from build123d import *

# Parameters (mm, degrees)
ESBO_O1_W                = 103
ESBO_O1_H                = 34
RESSALTO_EXTRUS_O1_DEPTH = 24
CORTE_EXTRUS_O1_DEPTH    = 0.5
FILETE1_R                = 2
SKETCH1_R                = 2.5
BOSS_EXTRUDE1_DEPTH      = 2


with BuildPart() as part:
    # Esboço1 → Ressalto-extrusão1 (new body)
    with BuildSketch(Plane.XY):
        Rectangle(ESBO_O1_W, ESBO_O1_H)
    extrude(amount=RESSALTO_EXTRUS_O1_DEPTH)

    # Esboço2 → Corte-extrusão1 (cut)
    with BuildSketch(Plane(origin=(51.5, 0, 0), x_dir=(0, 0, -1), z_dir=(1, 0, 0))):
        with BuildLine():
            Line((-4.5, 6), (-4.5, -6))
            ThreePointArc((-4.5, -6), (-12, -13.5), (-19.5, -6))
            Line((-19.5, -6), (-19.5, 6))
            ThreePointArc((-19.5, 6), (-12, 13.5), (-4.5, 6))
        make_face()
    corte_extrus_o1 = extrude(amount=-CORTE_EXTRUS_O1_DEPTH, mode=Mode.SUBTRACT)

    # Espelhar1: Corte-extrusão1 across plane
    add(corte_extrus_o1.mirror(Plane(origin=(0, 0, 0), x_dir=(0, 0, 1), z_dir=(1, 0, 0))), mode=Mode.SUBTRACT)

    # Filete1
    filete1_edges = [part.edges().sort_by_distance(p)[0] for p in [
        (-51.5, 0, 24),
        (0, -17, 24),
        (51.5, 0, 24),
        (0, -17, 0),
        (-51.5, 0, 0),
        (0, 17, 0),
        (51.5, 0, 0),
        (0, 17, 24),
        (51.5, -17, 12),
        (-51.5, -17, 12),
        (-51.5, 17, 12),
        (51.5, 17, 12),
    ]]
    fillet(filete1_edges, radius=FILETE1_R)

    # Sketch1 → Boss-Extrude1 (add)
    with BuildSketch(Plane.XY.offset(24)):
        Circle(SKETCH1_R)
    extrude(amount=BOSS_EXTRUDE1_DEPTH)


solid = part.part
Check sheet for the modelled part. Datum: model origin and axes. Units: mm. A direction names the side the tool comes from. Give positions to 0.01 mm unless a question says otherwise; leave off trailing zeros. Order: outer loops, then holes, each group sorted by start corner. A loop starts at its lowest first (then second) coordinate and runs counter-clockwise, first axis right, second up. Notation, with made-up numbers: M 0.25,19 L 46.25,19 A16 ccw 46.25,43 Z; hole C -34,-14.75 d6. An arc over 180 degrees is marked long. Answer as CSV lines item,"result". Start each with the question number.
Item 1: Gauge pin test, flat ends, axial feed: P1, Ø8, axis at x = -4.5, y = -6.5, coming from the +Z side; P2, Ø0.6, axis at x = -51.5, y = -1.5, coming from the +Z side; P3, Ø1, axis at x = 4, z = 23, coming from the -Y side. Record the tip position at first contact, or that the pin passes through.
Item 2: Cross-section at B-B on y = 0. Enter the section's corners in (x, z), plus the area to 3 significant figures.
Item 3: Cross-section at C-C on y = 11. Enter the section's corners in (x, z).
Item 4: Thickness scan on line 1 (X direction, y = 0, z = 15.5); line 2 (Z direction, x = 45, y = -8); line 3 (X direction, y = -7, z = 1.75). Record the ranges inside material, lowest first. Write a range as [from, to].
Item 5: Cross-section at A-A on x = -24. Enter the section's corners in (y, z), plus the area to 3 significant figures.
Item 6: Tool access check on faces 1 (the face through (-51.25, -13.5, 11.84)), 2 (the face through (51, 0, 12)), 3 (the face through (-50.93, -16.4, 12.14)). Record the directions out of +Z, -Z, +X, -X, +Y, -Y that give a thin tool (end or side, any length) a straight path to the whole face; none if there is none.
Item 7: Mould release check, pull along Z, two halves, no side actions. Record for faces 4 (the face through (51.5, 0, 3)), 5 (the face through (51.25, 13.5, 12.16)), 6 (the face through (-50.93, 0.21, 0.6)): +Z half, -Z half, draft (parallel to the pull), parting line (faces both ways), or undercut.
Established:
1,P1,"stops at z = 24"
1,P2,"stops at z = 23.05"
1,P3,"stops at y = -16.94"
2,outline,"M -51.5,2 A2 ccw -49.5,0 L 49.5,0 A2 ccw 51.5,2 L 51.5,4.5 L 51,4.5 L 51,19.5 L 51.5,19.5 L 51.5,22 A2 ccw 49.5,24 L 2.5,24 L 2.5,26 L -2.5,26 L -2.5,24 L -49.5,24 A2 ccw -51.5,22 L -51.5,19.5 L -51,19.5 L -51,4.5 L -51.5,4.5 Z"
2,area,"2,460 mm^2"
3,outline,"M -51.5,2 A2 ccw -49.5,0 L 49.5,0 A2 ccw 51.5,2 L 51.5,6.41 L 51,6.41 L 51,17.59 L 51.5,17.59 L 51.5,22 A2 ccw 49.5,24 L -49.5,24 A2 ccw -51.5,22 L -51.5,17.59 L -51,17.59 L -51,6.41 L -51.5,6.41 Z"
4,line 1,"x = [-51, 51]"
4,line 2,"z = [0, 24]"
4,line 3,"x = [-51.48, 51.48]"
5,outline,"M -17,2 A2 ccw -15,0 L 15,0 A2 ccw 17,2 L 17,22 A2 ccw 15,24 L -15,24 A2 ccw -17,22 Z"
5,area,"813 mm^2"
6,face 1,"-X"
6,face 2,"+X"
6,face 3,"+Z, -Z, -X, -Y"
7,face 4,"draft"
7,face 5,"undercut"
7,face 6,"-Z half"
